Verification items for the finished model (mm, model axes). A direction names the side the tool comes from. Give positions to 0.01 mm unless a question says otherwise; leave off trailing zeros. Loops run counter-clockwise (first coordinate to the right, second up) from the corner with the lowest first, then second, coordinate; pieces in that order, holes last. Notation, with made-up numbers: M 69,78.5 L 111,78.5 A21 cw 111,91.5 Z; hole C -5.5,-39 d9. An arc over 180 degrees is marked long. Answer in a Markdown table with one row per item.
```python
from build123d import *

# Parameters (mm, degrees)
BOSS_EXTRUDE1_DEPTH     = 3.8
CUT_EXTRUDE1_DEPTH      = 33.04999228
CUT_EXTRUDE2_DEPTH      = 30.761273573
CUT_EXTRUDE2_DEPTH_BACK = 30.761273573
SKETCH7_R               = 1.5
CUT_EXTRUDE3_DEPTH      = 8
SKETCH9_R               = 3.05
CUT_EXTRUDE4_DEPTH      = 8
SKETCH10_R              = 1.25
CUT_EXTRUDE5_DEPTH      = 33.0499924


with BuildPart() as part:
    # Sketch1 → Boss-Extrude1 (new body)
    with BuildSketch(Plane(origin=(0, 0, 0), x_dir=(1, 0, 0), z_dir=(0, 1, 0))):
        Polygon((-15.55, -17.05), (-15.55, 17.05), (-10.05, 17.05), (-7.75, 12.4), (7.75, 12.4), (10.05, 17.05), (15.55, 17.05), (15.55, -17.05), (10.05, -17.05), (7.75, -12.4), (-7.75, -12.4), (-10.05, -17.05), align=None)
    extrude(amount=BOSS_EXTRUDE1_DEPTH)

    # Revolve1: read off the stored shape, not the designer's step
    # Revolve1 outline → Revolve1 (revolve)
    with BuildSketch(Plane(origin=(-1.670959119, 0.964728697, 0), x_dir=(0.8660254037844398, -0.499999999999998, 0), z_dir=(0, 0, 1))):
        Polygon((10.200000298, -14.525), (10.200000248, 4.775000143), (3.79917118, 1.079479758), (0, 1.079479758), (0, -14.525), align=None)
    revolve(axis=Axis((-1.670959119, 0.964728697, 0), (0.499999999999998, 0.8660254037844398, 0)))

    # Sketch3 → Cut-Extrude1 (cut, through all)
    with BuildSketch(Plane(origin=(0, 3.8, 0), x_dir=(1, 0, 0), z_dir=(0, 1, 0))):
        Polygon((-10.05, 17.05), (-15.55, 17.05), (-15.55, -17.05), (-10.05, -17.05), (-7.75, -12.4), (7.75, -12.4), (10.05, -17.05), (15.55, -17.05), (15.55, 17.05), (10.05, 17.05), (7.75, 12.4), (-7.75, 12.4), align=None)
    extrude(amount=CUT_EXTRUDE1_DEPTH, mode=Mode.SUBTRACT)

    # Boundary-Cut1: read off the stored shape, not the designer's step
    # Boundary-Cut1: loft between two sections, ruled curve by curve
    boundary_cut1_from = [
        Edge.make_bspline([(-4.264195988, -14.310090618, 5.497330482), (-3.952600534, -14.489990338, 5.144451044), (-3.390059189, -14.814773735, 4.367149183), (-2.757568421, -15.17994245, 3.035429027), (-2.364627971, -15.406806725, 1.585508103), (-2.221728438, -15.489309808, 0.075173566), (-2.339233368, -15.421468305, -1.437931316), (-2.707711497, -15.208727358, -2.896270105), (-3.317731561, -14.85653211, -4.242306363), (-4.416065853, -14.222408511, -5.821756357), (-6.253782159, -13.161402507, -7.269581365), (-8.866989476, -11.652666559, -7.900430754), (-11.490387225, -10.138047163, -7.328308667), (-13.35210057, -9.063186462, -5.921916444), (-14.476778582, -8.413853309, -4.367433824), (-15.10932004, -8.048655327, -3.03533591), (-15.50227373, -7.821783409, -1.585450518), (-15.645207871, -7.739260344, -0.075222081), (-15.527690686, -7.807108923, 1.437904969), (-15.159193701, -8.019860756, 2.896296072), (-14.549188448, -8.372047453, 4.242316671), (-13.450871673, -9.006160938, 5.821729516), (-11.613084746, -10.067207715, 7.269617015), (-9.000025494, -11.575858178, 7.900380651), (-6.376366965, -13.090628136, 7.328435161), (-4.887386896, -13.95029118, 6.203089356), (-4.264195988, -14.310090618, 5.497330482)], [0, 0, 0, 0, 0.03125, 0.0625, 0.09375, 0.125, 0.15625, 0.1875, 0.21875, 0.25, 0.3125, 0.375, 0.4375, 0.5, 0.53125, 0.5625, 0.59375, 0.625, 0.65625, 0.6875, 0.71875, 0.75, 0.8125, 0.875, 0.9375, 1, 1, 1, 1], 3),
    ]
    boundary_cut1_to = [
        Edge.make_bspline([(3.535869827, 0, 6.0249567), (4.000260434, 0, 5.71827451), (4.874892388, 0, 5.020718912), (5.953015986, 0, 3.734542034), (6.720260155, 0, 2.238505144), (7.096013388, 0, 0.597243156), (7.030810986, 0, -1.085759731), (6.533226027, 0, -2.693977998), (5.66704479, 0, -4.133167867), (4.126269006, 0, -5.75895362), (1.680235047, 0, -7.172531093), (-1.628432874, 0, -7.851036071), (-4.989185483, 0, -7.528189152), (-7.581050356, 0, -6.415888298), (-9.330615811, 0, -5.020904789), (-10.408619135, 0, -3.734578971), (-11.176149314, 0, -2.238388975), (-11.55202821, 0, -0.597306131), (-11.48668895, 0, 1.0858282), (-10.988969574, 0, 2.693884042), (-10.123088416, 0, 4.133306502), (-8.582018083, 0, 5.758852747), (-6.136208886, 0, 7.172596545), (-2.827313809, 0, 7.85100057), (0.53292915, 0, 7.528284962), (2.607088614, 0, 6.63832108), (3.535869827, 0, 6.0249567)], [0, 0, 0, 0, 0.03125, 0.0625, 0.09375, 0.125, 0.15625, 0.1875, 0.21875, 0.25, 0.3125, 0.375, 0.4375, 0.5, 0.53125, 0.5625, 0.59375, 0.625, 0.65625, 0.6875, 0.71875, 0.75, 0.8125, 0.875, 0.9375, 1, 1, 1, 1], 3),
    ]
    boundary_cut1 = Solid(Shell([*[Face.make_surface_from_curves(boundary_cut1_from[k], boundary_cut1_to[k]) for k in range(1)], Face(Wire(boundary_cut1_from)), Face(Wire(boundary_cut1_to))]))
    add(boundary_cut1, mode=Mode.SUBTRACT)

    # Sketch7 → Cut-Extrude2 (cut, two sides: drawn at the far end of the back side and taken through both)
    with BuildSketch(Plane.XY.offset(-CUT_EXTRUDE2_DEPTH_BACK)):
        with Locations((-5.833459119, -6.24493279)):
            Circle(SKETCH7_R)
    extrude(amount=CUT_EXTRUDE2_DEPTH + CUT_EXTRUDE2_DEPTH_BACK, mode=Mode.SUBTRACT)

    # Sketch8 → Cut-Extrude3 (cut)
    with BuildSketch(Plane(origin=(0, 0, -17.05), x_dir=(-1, 0, 0), z_dir=(0, 0, -1))):
        Polygon((8.658459119, -4.613918279), (5.833459119, -2.982903769), (3.008459119, -4.613918279), (3.008459119, -7.8759473), (5.833459119, -9.50696181), (8.658459119, -7.8759473), align=None)
    extrude(amount=-CUT_EXTRUDE3_DEPTH, mode=Mode.SUBTRACT)

    # Sketch9 → Cut-Extrude4 (cut)
    with BuildSketch(Plane.XY.offset(17.05)):
        with Locations((-5.833459119, -6.24493279)):
            Circle(SKETCH9_R)
    extrude(amount=-CUT_EXTRUDE4_DEPTH, mode=Mode.SUBTRACT)

    # Sketch10 → Cut-Extrude5 (cut, through all)
    with BuildSketch(Plane(origin=(0, 3.8, 0), x_dir=(1, 0, 0), z_dir=(0, 1, 0))):
        with Locations(Location((-12.25, 13.4, 0), (0, 0, 270))):
            Circle(SKETCH10_R)
        with Locations(Location((-12.25, -13.4, 0), (0, 0, 270))):
            Circle(SKETCH10_R)
        with Locations(Location((12.25, -13.4, 0), (0, 0, 270))):
            Circle(SKETCH10_R)
        with Locations(Location((12.25, 13.4, 0), (0, 0, 270))):
            Circle(SKETCH10_R)
    extrude(amount=-CUT_EXTRUDE5_DEPTH, mode=Mode.SUBTRACT)


solid = part.part
```
Item 1: Tool access check on faces 1 (the flat face through (-8.916, 1.873, -14.758)), 2 (the flat face through (-15.55, 2, 0)), 3 (the flat face through (-4.441, -3.787, -9.633)), 4 (the flat face through (-2, 0, 0)). Record the directions out of +Z, -Z, +X, -X, +Y, -Y that give a thin tool (end or side, any length) a straight path to the whole face; none if there is none.
Reported:
| item | result |
|---|---|
| face 1 | -Z, +Y, -Y |
| face 2 | +Z, -Z, -X, +Y |
| face 3 | -Z |
| face 4 | none |
Item 2: Sectioned sample at A-A (x = 12.25). Record the cut outline in (y, z).
Reported:
| item | result |
|---|---|
| outline | M 0,-17.05 L 3.8,-17.05 L 3.8,-14.65 L 0,-14.65 Z; M 0,-12.15 L 3.8,-12.15 L 3.8,12.15 L 0,12.15 Z; M 0,14.65 L 3.8,14.65 L 3.8,17.05 L 0,17.05 Z |
Item 3: Sectioned sample at B-B (z = -13.4). Record the cut outline in (x, y).
Reported:
| item | result |
|---|---|
| outline | M -15.55,0 L -13.5,0 L -13.5,3.8 L -15.55,3.8 Z; M -11,0 L -8.24,0 L -8.24,3.8 L -11,3.8 Z; M 8.24,0 L 11,0 L 11,3.8 L 8.24,3.8 Z; M 13.5,0 L 15.55,0 L 15.55,3.8 L 13.5,3.8 Z |
Item 4: Sectioned sample at C-C (x = -5). State how many separate pieces and enclosed holes the cut face has, and give its area (3 significant figures).
Reported:
| item | result |
|---|---|
| separate pieces | 3 |
| enclosed holes | 0 |
| area | 147 mm^2 |
Item 5: Release check for a two-part mould opening along Y. For faces 5 (the flat face through (-10, -11, -8)), 6 (the flat face through (-5, -8, -9.05)), 7 (the flat face through (8.884, 1.873, -14.692)) record: released by +Y, released by -Y, zero draft, split by the parting line, or undercut.
Reported:
| item | result |
|---|---|
| face 5 | released by -Y |
| face 6 | undercut |
| face 7 | zero draft |
Item 6: Go/stop test with flat-tipped pins: pin 1 (1.5 mm diameter, centred on x = -7.5, y = -10, fed in from -Z); pin 2 (4 mm diameter, centred on x = 5.5, y = -0.5, fed in from -Z); pin 3 (5 mm diameter, centred on x = -5.83, y = -6.24, fed in from -Z). Record where each tip stops, or that it passes through.
Reported:
| item | result |
|---|---|
| pin 1 | stops at z = -10.2 |
| pin 2 | stops at z = -12.4 |
| pin 3 | stops at z = -9.05 |
Item 7: Scan lines: L1, parallel to X at y = 2.2, z = -13.4; L2, parallel to Z at x = -5.5, y = 1; L3, parallel to X at y = 2, z = 5.5. Record each from-to range of solid material in increasing order. Write a range as [from, to].
Reported:
| item | result |
|---|---|
| L1 | x = [-15.55, -13.5], [-11, -8.24], [8.24, 11], [13.5, 15.55] |
| L2 | z = [-12.4, 12.4] |
| L3 | x = [-15.55, 15.55] |
